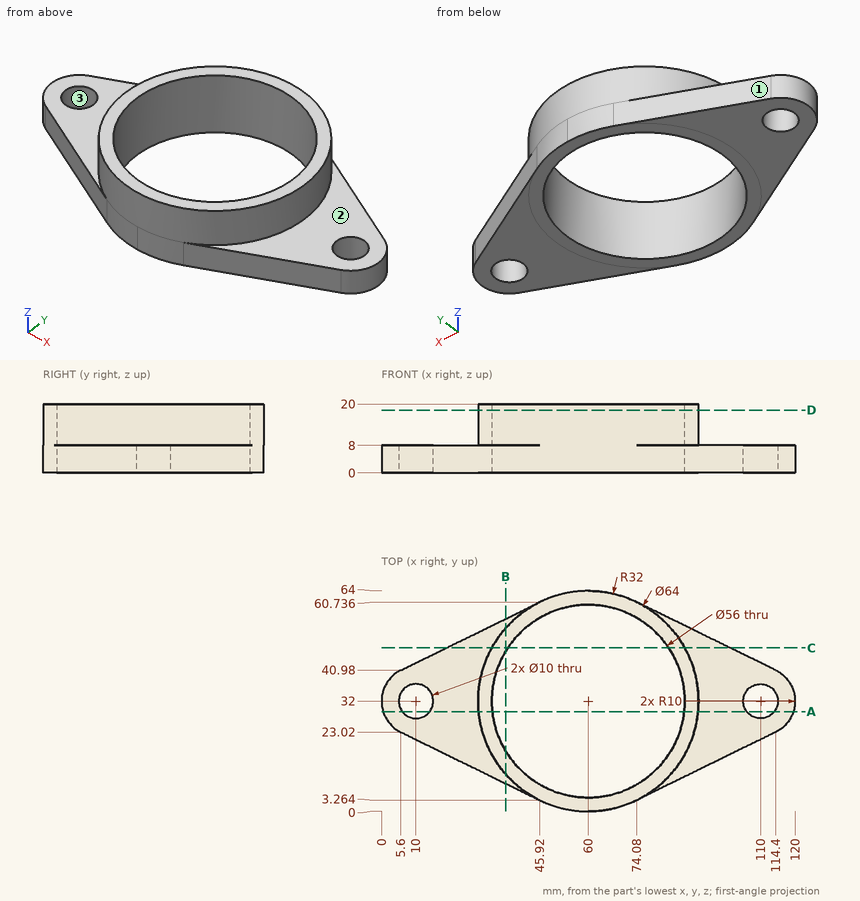
Verification items for this drawing (mm, ordinates from the low corner). Give positions to 0.01 mm unless a question says otherwise; leave off trailing zeros. Write each loop counter-clockwise with the first axis right and the second up, starting at its lowest first coordinate (ties: lowest second). Pieces come first, ordered by that corner, then holes.
1) Release check for a two-part mould opening along Y. For the marked faces 1, 2 and 3 record: released by +Y, released by -Y, zero draft, split by the parting line, or undercut.
Values follow:
face 1: released by +Y
face 2: zero draft
face 3: undercut
2) Cross-section at D-D (z = 18.25). Record the boundary of the cut face in (x, y).
Values follow:
outline: circle Ø64 at (60, 32); hole circle Ø56 at (60, 32)
3) Cross-section at A-A (y = 29). Record the boundary of the cut face in (x, z).
Values follow:
outline: (0.46, 0) - (6, 0) - (6, 8) - (0.46, 8) - close; (14, 0) - (32.16, 0) - (32.16, 20) - (28.14, 20) - (28.14, 8) - (14, 8) - close; (87.84, 0) - (106, 0) - (106, 8) - (91.86, 8) - (91.86, 20) - (87.84, 20) - close; (114, 0) - (119.54, 0) - (119.54, 8) - (114, 8) - close
4) Cross-section at C-C (y = 47.5). Record the boundary of the cut face in (x, z).
Values follow:
outline: (18.91, 0) - (36.68, 0) - (36.68, 20) - (32, 20) - (32, 8) - (18.91, 8) - close; (83.32, 0) - (101.09, 0) - (101.09, 8) - (88, 8) - (88, 20) - (83.32, 20) - close
5) Thickness scan on line 1 (Y direction, x = 60, z = 13); line 2 (X direction, y = 33, z = 3); line 3 (Z direction, x = 96, y = 26). Record the ranges inside material, lowest first.
Values follow:
line 1: y = 0 to 4, 60 to 64
line 2: x = 0.05 to 5.1, 14.9 to 32.02, 87.98 to 105.1, 114.9 to 119.95
line 3: z = 0 to 8
6) Go/stop test with flat-tipped pins: pin 1 Ø8 at (x, y) = (10, 32) entering from +Z; pin 2 Ø1.5 at (y, z) = (55, 17.5) entering from -X; pin 3 Ø1 at (x, y) = (102.5, 20.5) entering from +Z. Record where each tip stops, or that it passes through.
Values follow:
pin 1: passes through
pin 2: stops at x = 37
pin 3: stops at z = 8
7) Cross-section at B-B (x = 36). Record the boundary of the cut face in (y, z), plus the area to 3 significant figures.
Values follow:
outline: (8.12, 0) - (17.58, 0) - (17.58, 20) - (10.83, 20) - (10.83, 8) - (8.12, 8) - close; (46.42, 0) - (55.88, 0) - (55.88, 8) - (53.17, 8) - (53.17, 20) - (46.42, 20) - close
area: 313 mm2
